The model under review builds one solid part; all positions refer to its coordinate system, in mm. A direction names the side the tool comes from. Round coordinates to 2 decimals unless told otherwise and drop trailing zeros. Write each loop counter-clockwise with the first axis right and the second up, starting at its lowest first coordinate (ties: lowest second). Pieces come first, ordered by that corner, then holes. Notation, with made-up numbers: (54, 48.25) - (61, 48.25) arc R19 cw to (61, 74.25) - close; hole circle Ø8 at (83, 32). An arc over 180 degrees is marked (long way). Return JSON: item names as keys, results as strings.
from build123d import *

# Parameters (mm, degrees)
F3_ANGLE_BACK = 30
F3_ANGLE      = 60
F2_W          = 3.7940205075
F2_H          = 2.6295655407
F4_DEPTH      = 1


with BuildPart() as f3:
    # F0 (on Front) → F3 (revolve)
    with BuildSketch(Plane.XZ, mode=Mode.PRIVATE) as f3_sk:
        with BuildLine():
            Line((28.6788218176, -15.6407412676), (0, 25.3168609469))
            Line((0, 25.3168609469), (-28.6788218176, -15.6407412676))
            ThreePointArc((-28.6788218176, -15.6407412676), (0, -24.6831390531), (28.6788218176, -15.6407412676))
        make_face()
    revolve(f3_sk.sketch.rotate(Axis((3.0188281089, 0, 25.3168609469), (1, 0, 0)), -F3_ANGLE_BACK), axis=Axis((3.0188281089, 0, 25.3168609469), (1, 0, 0)), revolution_arc=F3_ANGLE)

    # F2 (on plane+point) → F4 (join, symmetric)
    with BuildSketch(Plane.XY.offset(25.3168609469)):
        with Locations((1.8970102537, 0)):
            Rectangle(F2_W, F2_H)
        with Locations((-1.8970102537, 0)):
            Rectangle(F2_W, F2_H)
    extrude(amount=F4_DEPTH, both=True)


solid = f3.part
(1) Mouldability with a two-part tool opening along Y and no side actions: class faces 1 (the flat face through (0, 1.315, 25)), 2 (the conical face through (14.494, -0.152, 4.618)), 3 (the flat face through (0, 0, 26.317)) as released by +Y, released by -Y, zero draft, split by the parting line, or undercut.
Filled in:
{"face 1": "released by +Y", "face 2": "undercut", "face 3": "zero draft"}
(2) Add section B-B (z = -19). Write out the cut boundary in (x, y), plus the area to 3 significant figures.
Filled in:
{"outline": "circle Ø46.3 at (0, 0)", "area": "1,680 mm2"}
(3) Wall thickness on line 1 (Z direction, x = 23, y = 16); line 2 (Z direction, x = 7, y = 4); line 3 (Y direction, x = 20, z = -4.5): over which ranges is each line inside the solid? List them lowest first.
Filled in:
{"line 1": "z = -16.1 to -3.37", "line 2": "z = -24.03 to 16.15", "line 3": "y = -17.21 to 17.21"}
(4) Add section C-C (x = -8). Write out the cut boundary in (y, z).
Filled in:
{"outline": "(-24.68, -17.43) arc R49.36 ccw to (24.68, -17.43) - (5.71, 15.42) arc R11.43 cw to (-5.71, 15.42) - close"}
(5) For faces 4 (the flat face through (3.794, 0, 25)), 5 (the flat face through (-3.794, 0, 25)), 6 (the flat face through (0, -1.315, 25)), list the 3-axis set-ups (+Z, -Z, +X, -X, +Y, -Y) from which the entire face can be reached by the end or side of a thin tool; tool diameter is ignored.
Filled in:
{"face 4": "+Z, +X, +Y, -Y", "face 5": "+Z, -X, +Y, -Y", "face 6": "+Z, +X, -X, -Y"}
(6) Clearance check with flat-ended pins moving along their axes: pin 1 Ø3 at (x, z) = (20, -2) entering from -Y; pin 2 Ø1.6 at (x, z) = (-2, 25) entering from -Y; pin 3 Ø5 at (y, z) = (-20, -15) entering from +X; pin 4 Ø8 at (y, z) = (13.5, 17.5) entering from -X. State where each tip first meets the part, or that it passes through.
Filled in:
{"pin 1": "stops at y = -16.64", "pin 2": "stops at y = -1.31", "pin 3": "stops at x = 26.33", "pin 4": "passes through"}
(7) Add section A-A (x = 13.5). Write out the cut boundary in (y, z).
Filled in:
{"outline": "(-24.07, -16.38) arc R48.14 ccw to (24.07, -16.38) - (9.64, 8.62) arc R19.28 cw to (-9.64, 8.62) - close"}
